Here's the drawing with two shaded views (mm, measured from the low corner). I have some questions. A direction names the side the tool comes from. Coordinates: 2 decimals unless noted, no trailing zeros. Order: outer loops, then holes, each group sorted by start corner. A loop starts at its lowest first (then second) coordinate and runs counter-clockwise, first axis right, second up. Notation, with made-up numbers: (-24.75, 67.5) - (1.25, 67.5) arc R8 cw to (1.25, 72.5) - close; hole circle Ø7 at (-31, -11.5). An arc over 180 degrees is marked (long way). Answer as a JSON object with one key per item and string values. Group by question number.
(1) Imagine slicing it at B-B, the plane y = 16. Write out the boundary of the cut face in (x, z), and give its area (3 significant figures).
(2) Will these pins go through, and if not, where does the flat tip stop? P1, Ø8, axis at x = 12, z = 27.5, coming from the +Y side; P2, Ø12, axis at x = 15, z = 7, coming from the -Y side (3 decimals); P3, Ø1, axis at y = 6.5, z = 21.5, coming from the -X side; P4, Ø8, axis at x = 6, z = 15.5, coming from the +Y side.
(3) Imagine slicing it at D-D, the plane y = 6. Write out the boundary of the cut face in (x, z), and give its area (3 significant figures).
(4) Which directions (+Z, -Z, +X, -X, +Y, -Y) give clear straight access to the entire face, cutting with the end or side of a thin tool? Please do the marked faces 1, 2 and 3.
(5) Please list where these lines run through material, in increasing order: probe 1 along Z at (x, y) = (5.5, 18); probe 2 along Y at (x, z) = (28, 20); probe 3 along Y at (x, z) = (13, 8.5).
(6) Imagine slicing it at C-C, the plane z = 4. Write out the boundary of the cut face in (x, y) (3 decimals), and give its area (3 significant figures).
(7) Imagine slicing it at A-A, the plane x = 9. Write out the boundary of the cut face in (y, z), and give its area (3 significant figures).
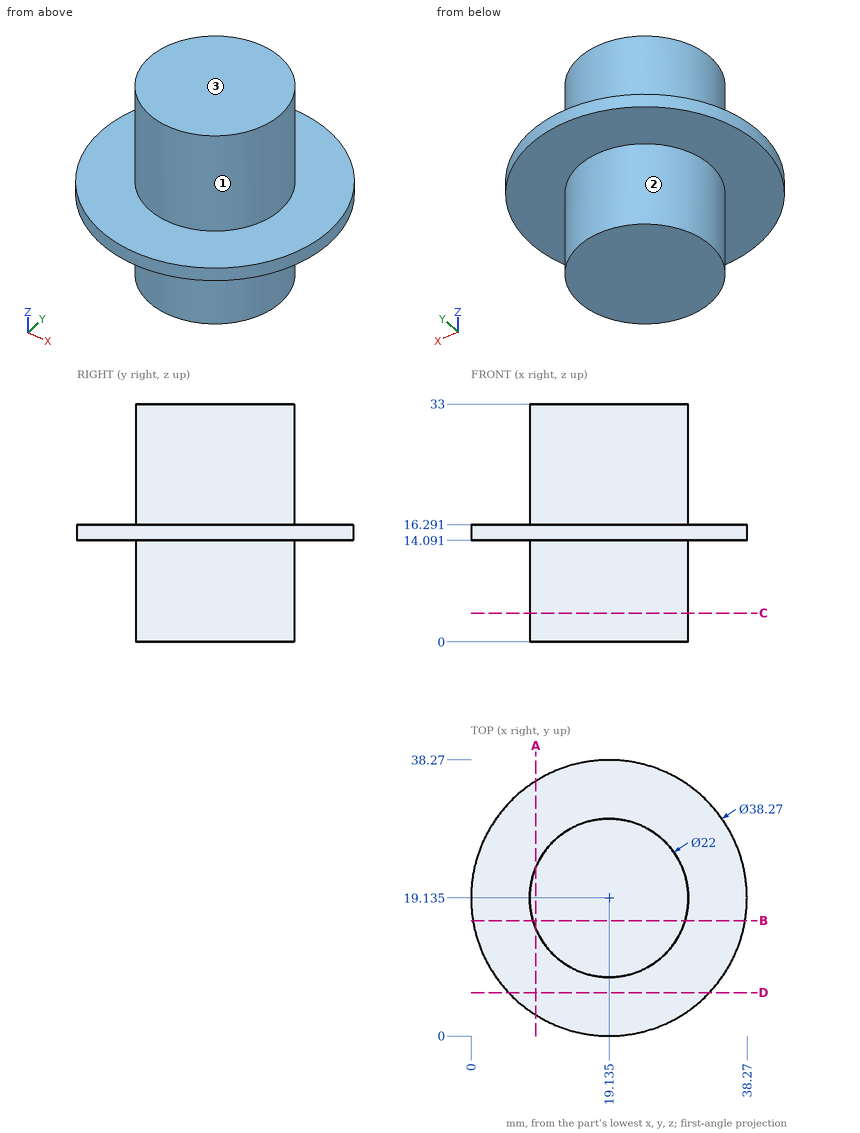
Result set:
{
 "1": {"outline": "(0.26, 14.09) - (8.59, 14.09) - (8.59, 0) - (29.68, 0) - (29.68, 14.09) - (38.01, 14.09) - (38.01, 16.29) - (29.68, 16.29) - (29.68, 33) - (8.59, 33) - (8.59, 16.29) - (0.26, 16.29) - close", "area": "733 mm^2"},
 "2": {"P1": "stops at y = 29.68", "P2": "stops at y = 8.135", "P3": "passes through", "P4": "stops at y = 35.95"},
 "3": {"outline": "(5.22, 14.09) - (33.05, 14.09) - (33.05, 16.29) - (5.22, 16.29) - close", "area": "61.2 mm^2"},
 "4": {"face 1": "+Z", "face 2": "-Z", "face 3": "+Z, +X, -X, +Y, -Y"},
 "5": {"probe 1": "z = 14.09 to 16.29", "probe 2": "y = 12.62 to 25.65", "probe 3": "y = 10 to 28.27"},
 "6": {"outline": "circle Ø22 at (19.135, 19.135)", "area": "380 mm^2"},
 "7": {"outline": "(2.9, 14.09) - (14.86, 14.09) - (14.86, 0) - (23.41, 0) - (23.41, 14.09) - (35.37, 14.09) - (35.37, 16.29) - (23.41, 16.29) - (23.41, 33) - (14.86, 33) - (14.86, 16.29) - (2.9, 16.29) - close", "area": "335 mm^2"}
}
